Geometry: final body of the model. Coordinates: model frame, mm. A direction names the side the tool comes from. Give positions to 0.01 mm unless a question says otherwise; leave off trailing zeros. Loops run counter-clockwise (first coordinate to the right, second up) from the corner with the lowest first, then second, coordinate; pieces in that order, holes last. Notation, with made-up numbers: M 85.25,-40 L 128.25,-40 A14 ccw 128.25,-19 Z; hole C 29.5,16.5 d3. An arc over 180 degrees is marked long. Put each result on its own line as item: value.
```python
from build123d import *

# Parameters (mm, degrees)
SKETCH_1_R               = 37.5
EXTRUDE_1_DEPTH          = 6
SKETCH_4_R               = 3
CUT_EXTRUDE_2_DEPTH      = 54.371340624
PATTERN_CIRCULAR_1_COUNT = 4
SKETCH_5_W               = 18
SKETCH_5_H               = 3
EXTRUDE_2_DEPTH          = 12
SKETCH_5_3_W             = 18
SKETCH_5_3_H             = 3
SKETCH_5_3_W_2           = 3
SKETCH_5_3_H_2           = 18
EXTRUDE_3_DEPTH          = 12
SKETCH_6_R               = 2.1
CUT_EXTRUDE_3_DEPTH      = 74.023968668
SKETCH_7_R               = 2.1
CUT_EXTRUDE_4_DEPTH      = 74.023968668


with BuildPart() as part:
    # Sketch 1 → Extrude 1 (new body)
    with BuildSketch(Plane(origin=(0, 0, 0), x_dir=(1, 0, 0), z_dir=(0, 1, 0))):
        with Locations(Location((0, 0, 0), (0, 0, 270))):
            Circle(SKETCH_1_R)
    extrude(amount=EXTRUDE_1_DEPTH)

    # Sketch 4 → Cut-Extrude 2 (cut, through all)
    with BuildSketch(Plane(origin=(0, 0, 0), x_dir=(1, 0, 0), z_dir=(0, 1, 0))):
        with Locations(Location((-17.67766953, 17.67766953, 0), (0, 0, 270))):
            Circle(SKETCH_4_R)
    cut_extrude_2 = extrude(amount=CUT_EXTRUDE_2_DEPTH, mode=Mode.SUBTRACT)

    # Pattern Circular 1: Cut-Extrude 2 ×4 about axis
    pattern_circular_1_axis = Axis((0, 0, 0), (0, 1, 0))
    for i in range(1, PATTERN_CIRCULAR_1_COUNT):
        add(cut_extrude_2.rotate(pattern_circular_1_axis, i * 360 / PATTERN_CIRCULAR_1_COUNT), mode=Mode.SUBTRACT)

    # Sketch 5 → Extrude 2 (add)
    with BuildSketch(Plane(origin=(0, 0, 0), x_dir=(-1, 0, 0), z_dir=(0, -1, 0))):
        with Locations((0, 22.5)):
            Rectangle(SKETCH_5_W, SKETCH_5_H)
    extrude_2 = extrude(amount=EXTRUDE_2_DEPTH)

    # Sketch 5_3 → Extrude 3 (add)
    with BuildSketch(Plane(origin=(0, 0, 0), x_dir=(-1, 0, 0), z_dir=(0, -1, 0))):
        with Locations((0, 22.5)):
            Rectangle(SKETCH_5_3_W, SKETCH_5_3_H)
        with Locations((22.5, 0)):
            Rectangle(SKETCH_5_3_W_2, SKETCH_5_3_H_2)
    extrude_3 = extrude(amount=EXTRUDE_3_DEPTH)

    # Mirror 3: Extrude 2 across plane
    add(extrude_2.mirror(Plane.XY))

    # Mirror 4: Extrude 3 across plane
    add(extrude_3.mirror(Plane(origin=(0, 0, 0), x_dir=(0, 0, 1), z_dir=(1, 0, 0))))

    # Sketch 6 → Cut-Extrude 3 (cut, through all)
    with BuildSketch(Plane.XY.offset(24)):
        with Locations((0, -6)):
            Circle(SKETCH_6_R)
    extrude(amount=-CUT_EXTRUDE_3_DEPTH, mode=Mode.SUBTRACT)

    # Sketch 7 → Cut-Extrude 4 (cut, through all)
    with BuildSketch(Plane(origin=(24, 0, 0), x_dir=(0, 0, -1), z_dir=(1, 0, 0))):
        with Locations((0, -6)):
            Circle(SKETCH_7_R)
    extrude(amount=-CUT_EXTRUDE_4_DEPTH, mode=Mode.SUBTRACT)


solid = part.part
```
Item 1: Line query: probe 1 along Y at (x, z) = (23.35, 0); probe 2 along Z at (x, y) = (0, -10); probe 3 along Y at (x, z) = (-26.5, 8.5). Output: solid intervals per line, ascending. Write a range as [from, to].
Output values:
probe 1: [-12, -8.1], [-3.9, 6]
probe 2: [-24, -21], [21, 24]
probe 3: [0, 6]
Item 2: Section B-B on z = 0. Output: boundary loops of the cut face in (x, y).
Output values:
outline: M -37.5,0 L -24,0 L -24,-3.9 L -21,-3.9 L -21,0 L 21,0 L 21,-3.9 L 24,-3.9 L 24,0 L 37.5,0 L 37.5,6 L -37.5,6 Z; M -24,-12 L -21,-12 L -21,-8.1 L -24,-8.1 Z; M 21,-12 L 24,-12 L 24,-8.1 L 21,-8.1 Z
Item 3: Set-up query: faces 4 (the flat face through (-21, -4.6, 2.1)), 5 (the flat face through (2.1, -4.6, 21)), 6 (the flat face through (2.1, -4.6, 24)), 7 (the flat face through (-9, -6, 22)), 8 (the flat face through (24, -4.6, 2.1)). Return all of +Z, -Z, +X, -X, +Y, -Y with unobstructed straight access to the full face (end or side cutting, diameter ignored); none if empty.
Output values:
face 4: +Z, -Z, -Y
face 5: +X, -X, -Y
face 6: +Z, +X, -X, -Y
face 7: +Z, -Z, -X, -Y
face 8: +Z, -Z, +X, -Y
Item 4: Section D-D on x = 29.5. Output: boundary loops of the cut face in (y, z), then the cut area to 3 significant figures.
Output values:
outline: M 0,-23.15 L 6,-23.15 L 6,23.15 L 0,23.15 Z
area: 278 mm²
Item 5: Section C-C on y = -6. Count the separate pieces of the cut face and the enclosed holes in it, then the cut area to 3 significant figures.
Output values:
separate pieces: 8
enclosed holes: 0
area: 166 mm²
Item 6: Pin query (flat end, axial travel): pin 1 Ø1.5 at (x, z) = (-4, -10) entering from -Y; pin 2 Ø9.5 at (x, y) = (0.5, -3) entering from +Z; pin 3 Ø6 at (y, z) = (-5, 3.5) entering from -X; pin 4 Ø6.5 at (x, y) = (0, -6) entering from -Z. Return the tip coordinate at first contact, or that it passes through.
Output values:
pin 1: y = 0
pin 2: z = 37.5
pin 3: x = -24
pin 4: z = -24
Item 7: Section A-A on x = 0. Output: boundary loops of the cut face in (y, z), then the cut area to 3 significant figures.
Output values:
outline: M -12,-24 L -8.1,-24 L -8.1,-21 L -12,-21 Z; M -12,21 L -8.1,21 L -8.1,24 L -12,24 Z; M -3.9,-24 L 0,-24 L 0,-37.5 L 6,-37.5 L 6,37.5 L 0,37.5 L 0,24 L -3.9,24 L -3.9,21 L 0,21 L 0,-21 L -3.9,-21 Z
area: 497 mm²
Item 8: Mould query, pull axis Z, two halves, no side actions, for faces 1 (the flat face through (-22, -6, -9)), 2 (the flat face through (22, -12, 0)), 3 (the cylindrical face through (18.328, 2.958, -20.606)). Classes: pulls with the +Z half, pulls with the -Z half, needs draft (parallel to the pull), parting line crosses it, or undercut.
Output values:
face 1: pulls with the -Z half
face 2: needs draft
face 3: undercut
